```python
from build123d import *

# Parameters (mm, degrees)
SKETCH_1_W          = 28
SKETCH_1_H          = 26
EXTRUDE_1_DEPTH     = 5
EXTRUDE_1_2_DEPTH   = 5
EXTRUDE_START       = 10
SKETCH_1_12_W       = 50
SKETCH_1_12_H       = 100
EXTRUDE_2_DEPTH     = 5
SKETCH_2_W          = 40
SKETCH_2_H          = 5
EXTRUDE_3_DEPTH     = 5
SKETCH_3_R          = 1.5
CUT_EXTRUDE_1_DEPTH = 131.38404815
SKETCH_3_3_R        = 2.25
CUT_EXTRUDE_2_DEPTH = 2
SKETCH_4_R          = 0.75
CUT_EXTRUDE_3_DEPTH = 4
SKETCH_5_R          = 31
CUT_EXTRUDE_4_DEPTH = 131.862523333
SKETCH_6_W          = 400
SKETCH_6_H          = 200
CUT_EXTRUDE_5_DEPTH = 131.862523333


with BuildPart() as part:
    # 草图1 → 凸台-拉伸1 (new body)
    with BuildSketch(Plane(origin=(0, 0, 0), x_dir=(1, 0, 0), z_dir=(0, 1, 0))):
        with Locations((106, 29.5)):
            Rectangle(SKETCH_1_W, SKETCH_1_H)
    extrude(amount=EXTRUDE_1_DEPTH)


with BuildPart() as body_2:
    # 草图1 → Extrude 1 2 (new body)
    with BuildSketch(Plane(origin=(0, 0, 0), x_dir=(1, 0, 0), z_dir=(0, 1, 0))):
        with Locations((106, -29.5)):
            Rectangle(SKETCH_1_W, SKETCH_1_H)
    extrude(amount=EXTRUDE_1_2_DEPTH)


with BuildPart() as body_3:
    # 草图1<12> → 凸台-拉伸2 (new body)
    with BuildSketch(Plane(origin=(0, 0, 0), x_dir=(1, 0, 0), z_dir=(0, 1, 0)).offset(EXTRUDE_START)):
        with Locations((25, 0)):
            Rectangle(SKETCH_1_12_W, SKETCH_1_12_H)
    extrude(amount=EXTRUDE_2_DEPTH)

    # 草图2 → 凸台-拉伸3 (add)
    with BuildSketch(Plane(origin=(50, 0, 0), x_dir=(0, 0, -1), z_dir=(1, 0, 0))):
        with Locations((30, 12.5)):
            Rectangle(SKETCH_2_W, SKETCH_2_H)
        with Locations((-30, 12.5)):
            Rectangle(SKETCH_2_W, SKETCH_2_H)
    extrude(amount=EXTRUDE_3_DEPTH)


    add(body_2.part)  # loft_5 joins it to this body
    # loft from a face of the part (loft_5)
    loft([body_3.faces().sort_by_distance((55, 12.5, 30))[0], body_3.faces().sort_by_distance((92, 2.5, 29.5))[0]])


    add(part.part)  # loft_6 joins it to this body
    # loft from a face of the part (loft_6)
    loft([body_3.faces().sort_by_distance((55, 12.5, -30))[0], body_3.faces().sort_by_distance((92, 2.5, -29.5))[0]])

    # 草图3 → 切除-拉伸1 (cut, through all)
    with BuildSketch(Plane(origin=(0, 5, 0), x_dir=(1, 0, 0), z_dir=(0, 1, 0))):
        with Locations(Location((113, 35.5, 0), (0, 0, 270))):
            Circle(SKETCH_3_R)
        with Locations(Location((99, 23.5, 0), (0, 0, 270))):
            Circle(SKETCH_3_R)
        with Locations(Location((113, -35.5, 0), (0, 0, 270))):
            Circle(SKETCH_3_R)
        with Locations(Location((99, -23.5, 0), (0, 0, 270))):
            Circle(SKETCH_3_R)
    extrude(amount=-CUT_EXTRUDE_1_DEPTH, mode=Mode.SUBTRACT)

    # 草图3<3> → 切除-拉伸2 (cut)
    with BuildSketch(Plane(origin=(0, 5, 0), x_dir=(1, 0, 0), z_dir=(0, 1, 0))):
        with Locations(Location((99, 23.5, 0), (0, 0, 270))):
            Circle(SKETCH_3_3_R)
        with Locations(Location((113, 35.5, 0), (0, 0, 270))):
            Circle(SKETCH_3_3_R)
        with Locations(Location((113, -35.5, 0), (0, 0, 270))):
            Circle(SKETCH_3_3_R)
        with Locations(Location((99, -23.5, 0), (0, 0, 270))):
            Circle(SKETCH_3_3_R)
    extrude(amount=-CUT_EXTRUDE_2_DEPTH, mode=Mode.SUBTRACT)

    # 草图4 → 切除-拉伸3 (cut)
    with BuildSketch(Plane(origin=(0, 15, 0), x_dir=(1, 0, 0), z_dir=(0, 1, 0))):
        with Locations((0, 36)):
            Circle(SKETCH_4_R)
        with Locations(Location((31.176914536, 18, 0), (0, 0, 270))):
            Circle(SKETCH_4_R)
        with Locations(Location((31.176914536, -18, 0), (0, 0, 270))):
            Circle(SKETCH_4_R)
        with Locations((0, -36)):
            Circle(SKETCH_4_R)
    extrude(amount=-CUT_EXTRUDE_3_DEPTH, mode=Mode.SUBTRACT)

    # 草图5 → 切除-拉伸4 (cut, through all)
    with BuildSketch(Plane(origin=(0, 15, 0), x_dir=(1, 0, 0), z_dir=(0, 1, 0))):
        Circle(SKETCH_5_R)
    extrude(amount=-CUT_EXTRUDE_4_DEPTH, mode=Mode.SUBTRACT)


with BuildPart() as body_2_2:
    # 镜向1: mirrored copy
    add(body_3.part.mirror(Plane(origin=(0, 0, 0), x_dir=(0, 0, 1), z_dir=(1, 0, 0))))

    # 草图6 → 切除-拉伸5 (cut, through all)
    with BuildSketch(Plane(origin=(0, 0, 0), x_dir=(0, 0, -1), z_dir=(1, 0, 0))):
        Rectangle(SKETCH_6_W, SKETCH_6_H)
    extrude(amount=-CUT_EXTRUDE_5_DEPTH, mode=Mode.SUBTRACT)


solid = body_3.part
```
The model under review builds one solid part; all positions refer to its coordinate system, in mm. A direction names the side the tool comes from. Give positions to 0.01 mm unless a question says otherwise; leave off trailing zeros. Write each loop counter-clockwise with the first axis right and the second up, starting at its lowest first coordinate (ties: lowest second). Pieces come first, ordered by that corner, then holes.
(1) Consider section B-B, the plane x = 16.5. Give the boundary of the cut face in (y, z).
(2) Consider section A-A, the plane x = 99. Give the boundary of the cut face in (y, z).
(3) To check wall thickness, follow L1, parallel to Z at x = 97, y = 1.5; L2, parallel to Y at x = 27, z = 20; L3, parallel to Y at x = 77, z = 41.5. State the ranges of each line that lie inside material, in increasing order.
(4) Tool access review of faces 1 (the flat face through (52, 12, 10)), 2 (the flat face through (33, 10, 1)), 3 (the cylindrical face through (96.804, 4.014, -23.988)), 4 (the flat face through (106, 5, 29)): name each direction out of +Z, -Z, +X, -X, +Y, -Y from which nothing blocks a thin tool from reaching the whole face with its end or side.
(5) Consider section D-D, the plane z = -5. Give the boundary of the cut face in (x, y), and give its area (3 significant figures).
(6) For P1, Ø5, axis at x = 76, z = -24, coming from the -Y side; P2, Ø2, axis at x = 114, z = -35.5, coming from the +Y side; P3, Ø5, axis at x = 113, z = 35.5, coming from the +Y side; P4, Ø1.5, axis at x = 28.5, y = 7.5, coming from the -Z side, all flat-tipped, find the tip position at first contact; note any pin that passes through.
(7) Consider section C-C, the plane y = 13.5. Give the number of separate pieces and of enclosed holes in the cut face, and give its area (3 significant figures).
(8) The part is to be moulded in two halves that separate along X. For faces 5 (the cylindrical face through (96.804, 4.014, 23.012)), 6 (the flat face through (106, 2, -16.5)), 7 (the flat face through (120, 2, 30)), say which applies: released by +X, released by -X, zero draft, split by the parting line, or undercut.
Returned:
1. outline: (10, -50) - (15, -50) - (15, -26.24) - (10, -26.24) - close; (10, 26.24) - (15, 26.24) - (15, 50) - (10, 50) - close
2. outline: (0, -42.5) - (5, -42.5) - (5, -25.75) - (3, -25.75) - (3, -25) - (0, -25) - close; (0, -22) - (3, -22) - (3, -21.25) - (5, -21.25) - (5, -16.5) - (0, -16.5) - close; (0, 16.5) - (5, 16.5) - (5, 21.25) - (3, 21.25) - (3, 22) - (0, 22) - close; (0, 25) - (3, 25) - (3, 25.75) - (5, 25.75) - (5, 42.5) - (0, 42.5) - close
3. L1: z = -42.5 to -16.5, 16.5 to 42.5
3. L2: y = 10 to 15
3. L3: y = 4.05 to 9.05
4. face 1: +X, +Y, -Y
4. face 2: +Z, -Z, -X, -Y
4. face 3: +Y
4. face 4: +Z, -Z, +X, +Y
5. outline: (30.59, 10) - (50, 10) - (50, 15) - (30.59, 15) - close
5. area: 97.0 mm2
6. P1: stops at y = 3.65
6. P2: stops at y = 3
6. P3: stops at y = 5
6. P4: passes through
7. separate pieces: 1
7. enclosed holes: 2
7. area: 4,320 mm2
8. face 5: undercut
8. face 6: zero draft
8. face 7: released by +X
